Design review of the part shown in the three views and the two pictorial views. Dimensions are in mm from the part's minimum x, y and z. Give positions to 0.01 mm unless a question says otherwise; leave off trailing zeros. Loops run counter-clockwise (first coordinate to the right, second up) from the corner with the lowest first, then second, coordinate; pieces in that order, holes last. Notation, with made-up numbers: (69, 38.5) - (100, 38.5) arc R35 ccw to (100, 77.5) - close; hole circle Ø5 at (41, 56). An arc over 180 degrees is marked (long way). Answer in a Markdown table with one row per item.
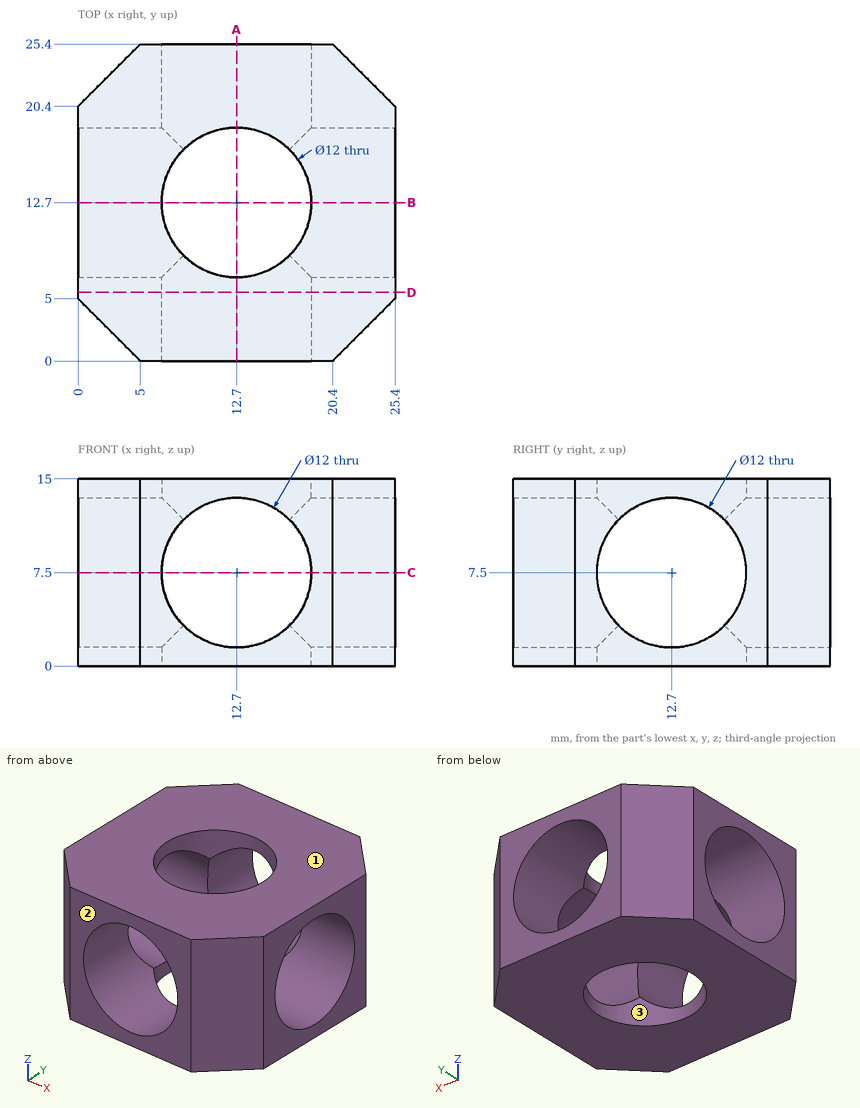
1. Mouldability with a two-part tool opening along Y and no side actions: class the marked faces 1, 2 and 3 as released by +Y, released by -Y, zero draft, split by the parting line, or undercut.
Values:
| item | result |
|---|---|
| face 1 | zero draft |
| face 2 | released by -Y |
| face 3 | undercut |
2. We need section D-D, the plane y = 5.5. Give the boundary of the cut face in (x, z).
Values:
| item | result |
|---|---|
| outline | (0, 0) - (25.4, 0) - (25.4, 15) - (0, 15) - close; hole circle Ø12 at (12.7, 7.5) |
3. Wall thickness on line 1 (X direction, y = 12.7, z = 1.1); line 2 (X direction, y = 17, z = 11.75): over which ranges is each line inside the solid? List them lowest first. Write a range as [from, to].
Values:
| item | result |
|---|---|
| line 1 | x = [0, 6.7], [18.7, 25.4] |
| line 2 | x = [0, 8.46], [16.94, 25.4] |
4. We need section C-C, the plane z = 7.5. Give the boundary of the cut face in (x, y).
Values:
| item | result |
|---|---|
| outline | (0, 5) - (5, 0) - (6.7, 0) - (6.7, 6.7) - (0, 6.7) - close; (0, 18.7) - (6.7, 18.7) - (6.7, 25.4) - (5, 25.4) - (0, 20.4) - close; (18.7, 0) - (20.4, 0) - (25.4, 5) - (25.4, 6.7) - (18.7, 6.7) - close; (18.7, 18.7) - (25.4, 18.7) - (25.4, 20.4) - (20.4, 25.4) - (18.7, 25.4) - close |
5. We need section A-A, the plane x = 12.7. Give the boundary of the cut face in (y, z).
Values:
| item | result |
|---|---|
| outline | (0, 0) - (6.7, 0) - (6.7, 1.5) - (0, 1.5) - close; (0, 13.5) - (6.7, 13.5) - (6.7, 15) - (0, 15) - close; (18.7, 0) - (25.4, 0) - (25.4, 1.5) - (18.7, 1.5) - close; (18.7, 13.5) - (25.4, 13.5) - (25.4, 15) - (18.7, 15) - close |
6. Clearance check with a flat-ended pin moving along its axis: pin 1 (3 mm diameter, centred on y = 22.5, z = 3, fed in from +X). State where the tip first meets the part, or that it passes through.
Values:
| item | result |
|---|---|
| pin 1 | stops at x = 24.8 |
